Input: part model. Units: mm. Frame: model coordinates. Face numbers are marked on the shaded views. A direction names the side the tool comes from. Give positions to 0.01 mm unless a question says otherwise; leave off trailing zeros. Write each loop counter-clockwise with the first axis right and the second up, starting at its lowest first coordinate (ties: lowest second). Pieces come first, ordered by that corner, then holes.
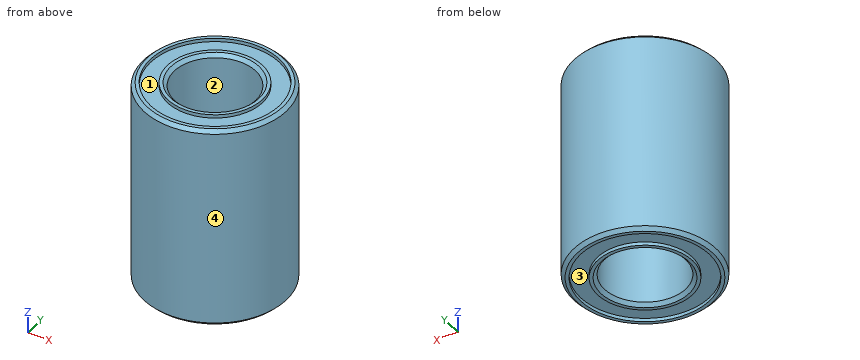
```python
from build123d import *

# Parameters (mm, degrees)
SKETCH1_R           = 10.5
SKETCH1_R_2         = 6
BOSS_EXTRUDE1_DEPTH = 30
SKETCH2_R           = 9.5
SKETCH2_R_2         = 7
CUT_EXTRUDE1_DEPTH  = 0.5
SKETCH3_R           = 9.5
SKETCH3_R_2         = 7
CUT_EXTRUDE2_DEPTH  = 0.5
CHAMFER1_SIZE       = 0.5


with BuildPart() as part:
    # Sketch1 → Boss-Extrude1 (new body)
    with BuildSketch(Plane.XY):
        Circle(SKETCH1_R)
        Circle(SKETCH1_R_2, mode=Mode.SUBTRACT)
    extrude(amount=BOSS_EXTRUDE1_DEPTH)

    # Sketch2 → Cut-Extrude1 (cut)
    with BuildSketch(Plane.XY.offset(30)):
        Circle(SKETCH2_R)
        Circle(SKETCH2_R_2, mode=Mode.SUBTRACT)
    extrude(amount=-CUT_EXTRUDE1_DEPTH, mode=Mode.SUBTRACT)

    # Sketch3 → Cut-Extrude2 (cut)
    with BuildSketch(Plane(origin=(0, 0, 0), x_dir=(-1, 0, 0), z_dir=(0, 0, -1))):
        Circle(SKETCH3_R)
        Circle(SKETCH3_R_2, mode=Mode.SUBTRACT)
    extrude(amount=-CUT_EXTRUDE2_DEPTH, mode=Mode.SUBTRACT)

    # Chamfer1
    chamfer1_edges = [part.edges().sort_by_distance(p)[0] for p in [
        (-10.5, 0, 0),
        (-10.5, 0, 30),
        (-6, 0, 0),
        (-6, 0, 30),
    ]]
    chamfer(chamfer1_edges, length=CHAMFER1_SIZE)


solid = part.part
```
Q1. Section C-C, the plane z = 13.5. Return the cut outline in (x, y), then the cut area to 3 significant figures.
Q2. Access query for the marked faces 1 and 2. Directions: +Z, -Z, +X, -X, +Y, -Y. A direction counts if a zero-diameter tool reaches every point of the face in a straight line with its end or side. Return the directions, or none.
Q3. Mould query, pull axis X, two halves, no side actions, for the marked faces 3 and 4. Classes: +X half, -X half, draft (parallel to the pull), parting line (faces both ways), or undercut.
Q4. Material intervals for line 1 along Y through (x, z) = (0, 29.85); line 2 along Y through (x, z) = (0, 29.7); line 3 along Y through (x, z) = (0, 23.75), sorted ascending.
Q5. Pin query (flat end, axial travel): pin 1 (9.5 mm diameter, centred on x = 0.5, y = 1, fed in from -Z); pin 2 (6 mm diameter, centred on y = -6.5, z = 17, fed in from -X); pin 3 (3 mm diameter, centred on y = -4.5, z = 3.5, fed in from -X); pin 4 (1 mm diameter, centred on x = -2.5, z = 9, fed in from -Y). Return the tip coordinate at first contact, or that it passes through.
Solutions:
1. outline: circle Ø21 at (0, 0); hole circle Ø12 at (0, 0)
1. area: 233 mm2
2. face 1: +Z
2. face 2: +Z, -Z
3. face 3: undercut
3. face 4: parting line
4. line 1: y = -10.15 to -9.5, -7 to -6.35, 6.35 to 7, 9.5 to 10.15
4. line 2: y = -10.3 to -9.5, -7 to -6.2, 6.2 to 7, 9.5 to 10.3
4. line 3: y = -10.5 to -6, 6 to 10.5
5. pin 1: passes through
5. pin 2: stops at x = -9.9
5. pin 3: stops at x = -10.06
5. pin 4: stops at y = -10.31
